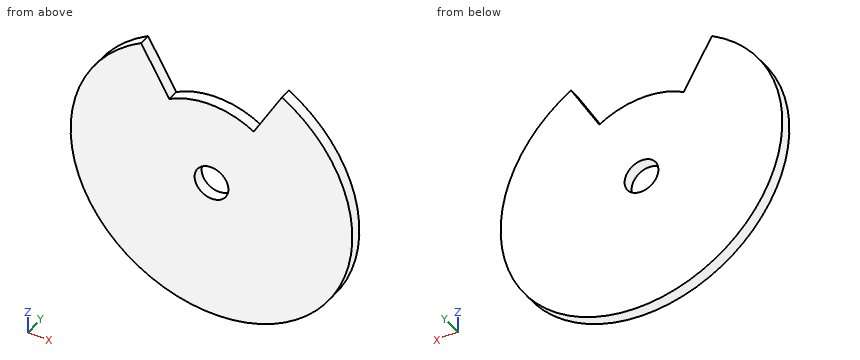
```python
from build123d import *

# Parameters (mm, degrees)
SKETCH_1_R      = 3
EXTRUDE_1_DEPTH = 2


with BuildPart() as part:
    # Эскиз1 → Бобышка-Вытянуть1 (new body)
    with BuildSketch(Plane(origin=(0, 0, 0), x_dir=(1, 0, 0), z_dir=(0, 1, 0))):
        with BuildLine():
            ThreePointArc((-7.5, -12.990381057), (0, -15), (7.5, -12.990381057))
            Line((7.5, -12.990381057), (12.5, -21.650635095))
            ThreePointArc((12.5, -21.650635095), (0, 25), (-12.5, -21.650635095))
            Line((-12.5, -21.650635095), (-7.5, -12.990381057))
        make_face()
        Circle(SKETCH_1_R, mode=Mode.SUBTRACT)
    extrude(amount=EXTRUDE_1_DEPTH)


solid = part.part
```
Can you work these out from the model? Positions are in its coordinate system, mm. Round coordinates to 2 decimals unless told otherwise and drop trailing zeros. Loops run counter-clockwise (first coordinate to the right, second up) from the corner with the lowest first, then second, coordinate; pieces in that order, holes last. Notation, with made-up numbers: M 31.25,39.5 L 54.25,39.5 A33 ccw 54.25,69.5 Z; hole C 35,-37 d4. An arc over 180 degrees is marked long. Answer as a JSON object with one key per item and string values. Group by question number.
Q1. Please list where these lines run through material, in increasing order: L1, parallel to Z at x = 0, y = 1; L2, parallel to X at y = 1, z = 1.5; L3, parallel to X at y = 1.2, z = 15.5.
Q2. Imagine slicing it at D-D, the plane z = -13.5. Please give me the cut outline in (x, y).
Q3. Imagine slicing it at B-B, the plane z = 0. Please give me the cut outline in (x, y), then the cut area to 3 significant figures.
Q4. Imagine slicing it at C-C, the plane x = 16. Please give me the cut outline in (y, z).
Q5. Imagine slicing it at A-A, the plane x = 0. Please give me the cut outline in (y, z), then the cut area to 3 significant figures.
Findings:
{
 "1": {"L1": "z = -25 to -3, 3 to 15", "L2": "x = -24.95 to -2.6, 2.6 to 24.95", "L3": "x = -19.62 to -8.95, 8.95 to 19.62"},
 "2": {"outline": "M -21.04,0 L 21.04,0 L 21.04,2 L -21.04,2 Z"},
 "3": {"outline": "M -25,0 L -3,0 L -3,2 L -25,2 Z; M 3,0 L 25,0 L 25,2 L 3,2 Z", "area": "88.0 mm2"},
 "4": {"outline": "M 0,-19.21 L 2,-19.21 L 2,19.21 L 0,19.21 Z"},
 "5": {"outline": "M 0,-25 L 2,-25 L 2,-3 L 0,-3 Z; M 0,3 L 2,3 L 2,15 L 0,15 Z", "area": "68.0 mm2"}
}
